Autodesk Inventor part; units mm, degrees
ref_plane "YZ Plane" through (0, 0, 0) normal (1, 0, 0) x (0, 1, 0)
ref_plane "XZ Plane" through (0, 0, 0) normal (0, 1, 0) x (-1, 0, 0)
ref_plane "XY Plane" through (0, 0, 0) normal (0, 0, 1) x (1, 0, 0)
sketch "Sketch1" plane through (0, 0, 0) normal (0, 1, 0) x (-1, 0, 0)
  line L0 (0, 0) -> (180, 0)
  line L1 (180, 0) -> (180, -180)
  line L2 (180, -180) -> (0, -180)
  line L3 (0, -180) -> (0, 0)
  circle A0 centre (90, -90) radius 18.75
  circle A1 centre (90, -51.675) radius 3.2
  line L4 (90, -51.675) -> (90, -90) construction
  point P0 (180, -90)
  point P1 (90, -180)
  dimension "d0" = 180
  dimension "d1" = 180
  dimension "d2" = 37.5
  dimension "d3" = 0
  dimension "d4" = 0
  dimension "d5" = 6.4
  dimension "d6" = 38.325
extrude "Extrusion1" add sketch "Sketch1" along normal blind 9.5813
properties part number "base_plate" material "Pine"
Input: part model. Units: mm. Frame: model coordinates. Give positions to 0.01 mm unless a question says otherwise; leave off trailing zeros. Loops run counter-clockwise (first coordinate to the right, second up) from the corner with the lowest first, then second, coordinate; pieces in that order, holes last. Notation, with made-up numbers: (-33, 22.25) - (25, 22.25) arc R33 cw to (25, 56.25) - close; hole circle Ø5 at (27.5, -24.75). An arc over 180 degrees is marked (long way). Use CSV: the item, a comma, the result in double quotes. Start each with the question number.
Item 1: Section A-A on x = -90. Return loops of the section in (y, z) (3 decimals).
Item 2: Mould query, pull axis Z, two halves, no side actions, for faces 1 (the cylindrical face through (-89.31, 4.72, -48.55)), 2 (the flat face through (0, 5, -91)), 3 (the flat face through (-91, 5, -180)). Classes: pulls with the +Z half, pulls with the -Z half, needs draft (parallel to the pull), parting line crosses it, or undercut.
Item 3: Line query: line 1 (Z direction, x = -90, y = 4.5) (3 decimals); line 2 (X direction, y = 1.25, z = -52); line 3 (Z direction, x = -75, y = 7). Output: solid intervals per line, ascending.
Item 4: Contact query for flat-ended pins moving along their axis: P1, Ø6, axis at x = -152.5, z = -63.5, coming from the -Y side; P2, Ø4, axis at x = -90, z = -51.675, coming from the +Y side. Output: stop coordinate, or through.
Item 5: Section B-B on z = -90. Return loops of the section in (x, y), then the cut area to 3 significant figures.
Ans:
1,outline,"(0, -180) - (9.581, -180) - (9.581, -108.75) - (0, -108.75) - close; (0, -71.25) - (9.581, -71.25) - (9.581, -54.875) - (0, -54.875) - close; (0, -48.475) - (9.581, -48.475) - (9.581, 0) - (0, 0) - close"
2,face 1,"undercut"
2,face 2,"needs draft"
2,face 3,"pulls with the -Z half"
3,line 1,"z = -180 to -108.75, -71.25 to -54.875, -48.475 to 0"
3,line 2,"x = -180 to -93.18, -86.82 to 0"
3,line 3,"z = -180 to -101.25, -78.75 to 0"
4,P1,"stops at y = 0"
4,P2,"passes through"
5,outline,"(-180, 0) - (-108.75, 0) - (-108.75, 9.58) - (-180, 9.58) - close; (-71.25, 0) - (0, 0) - (0, 9.58) - (-71.25, 9.58) - close"
5,area,"1,370 mm2"
